Source: CAD feature listing. Evaluate the final solid. Frame: model axes, mm. Round coordinates to 2 decimals unless told otherwise and drop trailing zeros. Order: outer loops, then holes, each group sorted by start corner. A loop starts at its lowest first (then second) coordinate and runs counter-clockwise, first axis right, second up. Notation, with made-up numbers: (-26, 53) -> (9, 53) arc R26 cw to (9, 87) -> close; hole circle Ø11 at (44.5, 31.25). An arc over 180 degrees is marked (long way). Answer as CSV lines item,"result".
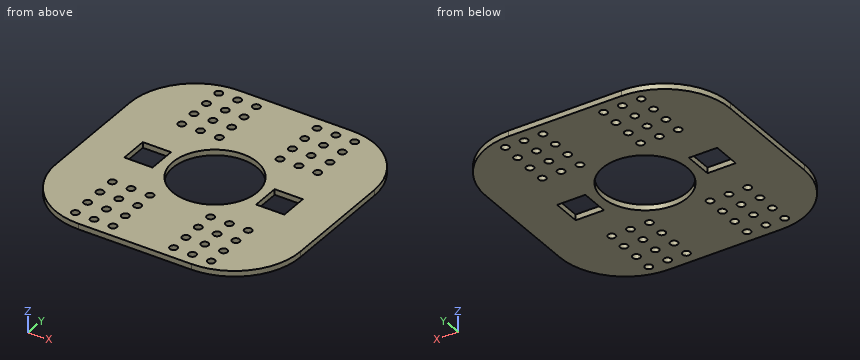
from build123d import *

# Parameters (mm, degrees)
SKETCH_1_W          = 130
SKETCH_1_H          = 130
SKETCH_1_R          = 22.5
EXTRUDE_1_DEPTH     = 3
FILLET_1_R          = 35
SKETCH_5_R          = 2
SKETCH_5_W          = 15
SKETCH_5_H          = 15
CUT_EXTRUDE_2_DEPTH = 13


with BuildPart() as part:
    # 草图1 → 凸台-拉伸1 (new body)
    with BuildSketch(Plane.XY):
        Rectangle(SKETCH_1_W, SKETCH_1_H)
        Circle(SKETCH_1_R, mode=Mode.SUBTRACT)
    extrude(amount=-EXTRUDE_1_DEPTH)

    # 圆角1
    fillet_1_edges = [part.edges().sort_by_distance(p)[0] for p in [
        (65, -65, -1.5),
        (-65, -65, -1.5),
        (-65, 65, -1.5),
        (65, 65, -1.5),
    ]]
    fillet(fillet_1_edges, radius=FILLET_1_R)

    # 草图5 → 切除-拉伸2 (cut)
    with BuildSketch(Plane(origin=(0, 0, -3), x_dir=(-1, 0, 0), z_dir=(0, 0, -1))):
        with Locations((36.119111303, 58.196758832)):
            Circle(SKETCH_5_R)
        with Locations((36.119111303, 48.196758832)):
            Circle(SKETCH_5_R)
        with Locations((36.119111303, 38.196758832)):
            Circle(SKETCH_5_R)
        with Locations((-36.119111303, -58.196758832)):
            Circle(SKETCH_5_R)
        with Locations((16.119111303, 48.196758832)):
            Circle(SKETCH_5_R)
        with Locations((16.119111303, 38.196758832)):
            Circle(SKETCH_5_R)
        with Locations((16.119111303, 28.196758832)):
            Circle(SKETCH_5_R)
        with Locations((26.119111303, 58.196758832)):
            Circle(SKETCH_5_R)
        with Locations((16.119111303, -48.196758832)):
            Circle(SKETCH_5_R)
        with Locations((26.119111303, -28.196758832)):
            Circle(SKETCH_5_R)
        with Locations((36.119111303, 28.196758832)):
            Circle(SKETCH_5_R)
        with Locations((26.119111303, 48.196758832)):
            Circle(SKETCH_5_R)
        with Locations((26.119111303, 38.196758832)):
            Circle(SKETCH_5_R)
        with Locations((26.119111303, 28.196758832)):
            Circle(SKETCH_5_R)
        with Locations((16.119111303, 58.196758832)):
            Circle(SKETCH_5_R)
        with Locations((16.119111303, -58.196758832)):
            Circle(SKETCH_5_R)
        with Locations((26.119111303, -58.196758832)):
            Circle(SKETCH_5_R)
        with Locations((16.119111303, -28.196758832)):
            Circle(SKETCH_5_R)
        with Locations((16.119111303, -38.196758832)):
            Circle(SKETCH_5_R)
        with Locations((36.119111303, -38.196758832)):
            Circle(SKETCH_5_R)
        with Locations((36.119111303, -48.196758832)):
            Circle(SKETCH_5_R)
        with Locations((36.119111303, -58.196758832)):
            Circle(SKETCH_5_R)
        with Locations((-36.119111303, -48.196758832)):
            Circle(SKETCH_5_R)
        with Locations((-36.119111303, -38.196758832)):
            Circle(SKETCH_5_R)
        with Locations((-16.119111303, -38.196758832)):
            Circle(SKETCH_5_R)
        with Locations((-16.119111303, -28.196758832)):
            Circle(SKETCH_5_R)
        with Locations((-26.119111303, -58.196758832)):
            Circle(SKETCH_5_R)
        with Locations((26.119111303, -38.196758832)):
            Circle(SKETCH_5_R)
        with Locations((26.119111303, -48.196758832)):
            Circle(SKETCH_5_R)
        with Locations((36.119111303, -28.196758832)):
            Circle(SKETCH_5_R)
        with Locations((-36.119111303, -28.196758832)):
            Circle(SKETCH_5_R)
        with Locations((-26.119111303, -48.196758832)):
            Circle(SKETCH_5_R)
        with Locations((-26.119111303, -38.196758832)):
            Circle(SKETCH_5_R)
        with Locations((-26.119111303, -28.196758832)):
            Circle(SKETCH_5_R)
        with Locations((-16.119111303, -48.196758832)):
            Circle(SKETCH_5_R)
        with Locations((-16.119111303, 28.196758832)):
            Circle(SKETCH_5_R)
        with Locations((-16.119111303, 38.196758832)):
            Circle(SKETCH_5_R)
        with Locations((-16.119111303, 48.196758832)):
            Circle(SKETCH_5_R)
        with Locations((-26.119111303, 28.196758832)):
            Circle(SKETCH_5_R)
        with Locations((-26.119111303, 38.196758832)):
            Circle(SKETCH_5_R)
        with Locations((-36.119111303, 38.196758832)):
            Circle(SKETCH_5_R)
        with Locations((-36.119111303, 48.196758832)):
            Circle(SKETCH_5_R)
        with Locations((-36.119111303, 58.196758832)):
            Circle(SKETCH_5_R)
        with Locations((-16.119111303, -58.196758832)):
            Circle(SKETCH_5_R)
        with Locations((-16.119111303, 58.196758832)):
            Circle(SKETCH_5_R)
        with Locations((-26.119111303, 58.196758832)):
            Circle(SKETCH_5_R)
        with Locations((-26.119111303, 48.196758832)):
            Circle(SKETCH_5_R)
        with Locations((-36.119111303, 28.196758832)):
            Circle(SKETCH_5_R)
        with Locations((35.031984266, -1.155156202)):
            Rectangle(SKETCH_5_W, SKETCH_5_H)
        with Locations((-35.031984266, -1.155156202)):
            Rectangle(SKETCH_5_W, SKETCH_5_H)
    extrude(amount=-CUT_EXTRUDE_2_DEPTH, mode=Mode.SUBTRACT)


solid = part.part
1. Pin query (flat end, axial travel): pin 1 (5 mm diameter, centred on x = 16.12, y = 58.2, fed in from +Z); pin 2 (3.5 mm diameter, centred on x = -16.12, y = 28.2, fed in from +Z). Return the tip coordinate at first contact, or that it passes through.
Results below:
pin 1,"z = 0"
pin 2,"through"
2. Section query B-B on y = 0. Return loops of the section in (x, z).
Results below:
outline,"(-65, -3) -> (-42.53, -3) -> (-42.53, 0) -> (-65, 0) -> close; (-27.53, -3) -> (-22.5, -3) -> (-22.5, 0) -> (-27.53, 0) -> close; (22.5, -3) -> (27.53, -3) -> (27.53, 0) -> (22.5, 0) -> close; (42.53, -3) -> (65, -3) -> (65, 0) -> (42.53, 0) -> close"
3. Section query A-A on x = 0. Return loops of the section in (y, z).
Results below:
outline,"(-65, -3) -> (-22.5, -3) -> (-22.5, 0) -> (-65, 0) -> close; (22.5, -3) -> (65, -3) -> (65, 0) -> (22.5, 0) -> close"
4. Section query C-C on y = 20. Return loops of the section in (x, z).
Results below:
outline,"(-65, -3) -> (-10.31, -3) -> (-10.31, 0) -> (-65, 0) -> close; (10.31, -3) -> (65, -3) -> (65, 0) -> (10.31, 0) -> close"
5. Section query D-D on z = -1.95. Give the number of separate pieces and of enclosed holes in the cut face, and give its area (3 significant figures).
Results below:
separate pieces,"1"
enclosed holes,"51"
area,"13,200 mm2"
6. Line query: L1, parallel to X at y = -1, z = -0.3; L2, parallel to Y at x = 1, z = -0.75; L3, parallel to X at y = 4, z = -0.5. Output: solid intervals per line, ascending. Write a range as [from, to].
Results below:
L1,"[-65, -42.53], [-27.53, -22.48], [22.48, 27.53], [42.53, 65]"
L2,"[-65, -22.48], [22.48, 65]"
L3,"[-65, -42.53], [-27.53, -22.14], [22.14, 27.53], [42.53, 65]"
